from build123d import *

# Parameters (mm, degrees)
F1_DEPTH = 25
F3_DEPTH = 75
F4_W     = 5.629124
F4_H     = 6
F5_DEPTH = 35
F6_W     = 6.780945
F6_H     = 9.562873
F7_DEPTH = 3
F8_W     = 2
F8_H     = 9.562873
F9_DEPTH = 6


with BuildPart() as f1:
    # F0 (on Top) → F1 (new body)
    with BuildSketch(Plane.XY):
        with BuildLine():
            Line((-4.536292, 28.185949), (-55.529496, 19.979021))
            ThreePointArc((-55.529496, 19.979021), (-73.186468, 0), (-55.529496, -19.979021))
            Line((-55.529496, -19.979021), (-4.536292, -28.185949))
            ThreePointArc((-4.536292, -28.185949), (28.548654, 0), (-4.536292, 28.185949))
        make_face()
    extrude(amount=F1_DEPTH)

    # F2 (on face) → F3 (join)
    with BuildSketch(Plane.XY.offset(25)):
        Polygon((-10, 4.142136), (-10, -4.142136), (-4.142136, -10), (4.142136, -10), (10, -4.142136), (10, 4.142136), (4.142136, 10), (-4.142136, 10), align=None)
    extrude(amount=F3_DEPTH)

    # F4 (on face) → F5 (join)
    with BuildSketch(Plane.YZ.offset(10)):
        with Locations((-0.144606, 92.806667)):
            Rectangle(F4_W, F4_H)
    extrude(amount=F5_DEPTH)

    # F6 (on Front) → F7 (join, symmetric)
    with BuildSketch(Plane.XZ):
        with Locations((46.465266, 93.107711)):
            Rectangle(F6_W, F6_H)
    extrude(amount=F7_DEPTH, both=True)

    # F8 (on face) → F9 (cut)
    with BuildSketch(Plane.YZ.offset(49.855739)):
        with Locations((-0.098561, 93.107711)):
            Rectangle(F8_W, F8_H)
    extrude(amount=-F9_DEPTH, mode=Mode.SUBTRACT)


solid = f1.part
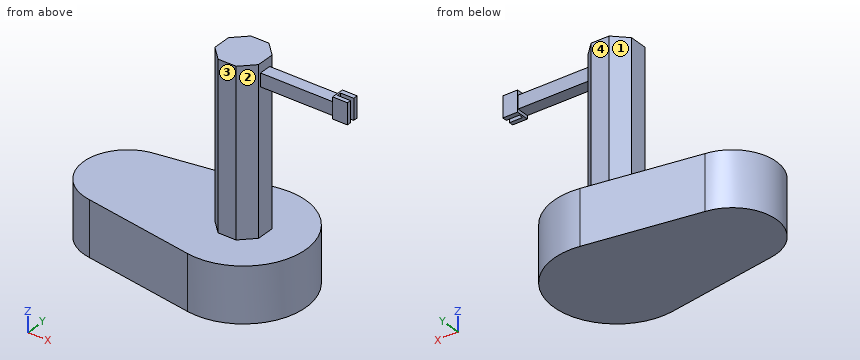
Build history of the part. All positions in model axes, mm. Face numbers are marked on the shaded views. A direction names the side the tool comes from. Give positions to 0.01 mm unless a question says otherwise; leave off trailing zeros. Order: outer loops, then holes, each group sorted by start corner. A loop starts at its lowest first (then second) coordinate and runs counter-clockwise, first axis right, second up. Notation, with made-up numbers: M 54,23 L 69,23 A19 ccw 69,39 Z; hole C 72,8 d10. An arc over 180 degrees is marked long. Use one line per item in the form item = value.
1) Drop flat-ended pins along their axis: pin 1 (4 mm diameter, centred on y = 1.5, z = 57.5, fed in from +X); pin 2 (9 mm diameter, centred on y = 1, z = 80.5, fed in from -X); pin 3 (6.5 mm diameter, centred on x = 32, z = 93, fed in from -Y). Give the stop position or say it passes through.
Calculated:
pin_1 = 10
pin_2 = -10
pin_3 = -2.96
2) Saw through at B-B (z = 29.5). Give the cut face in (x, y).
Calculated:
outline = M -10,-4.14 L -4.14,-10 L 4.14,-10 L 10,-4.14 L 10,4.14 L 4.14,10 L -4.14,10 L -10,4.14 Z
3) Tool access for the marked faces 1, 2, 3 and 4: list every direction of +Z, -Z, +X, -X, +Y, -Y with a clear straight run to the whole face (end or side of a thin tool).
Calculated:
face_1 = +Z, -X, +Y
face_2 = +Z, +X, -Y
face_3 = +Z, +X, -X, -Y
face_4 = +Z, +X, -X, +Y
4) Probe probe 1 along Z at (x, y) = (2.5, 12); probe 2 along Y at (x, z) = (-2, 95.5); probe 3 along Y at (x, z) = (44, 90.5). List the from-to ranges inside material, lowest first.
Calculated:
probe_1 = 0 to 25
probe_2 = -10 to 10
probe_3 = -3 to -1.1, 0.9 to 3
5) Saw through at C-C (y = -22). Give the cut face in (x, z), plus the area to 3 significant figures.
Calculated:
outline = M -42.97,0 L 18.19,0 L 18.19,25 L -42.97,25 Z
area = 1,530 mm2
6) Saw through at D-D (x = 34). Give the cut face in (y, z), plus the area to 3 significant figures.
Calculated:
outline = M -2.96,89.81 L 2.67,89.81 L 2.67,95.81 L -2.96,95.81 Z
area = 33.8 mm2
7) Saw through at A-A (x = 0). Give the cut face in (y, z), plus the area to 3 significant figures.
Calculated:
outline = M -28.55,0 L 28.55,0 L 28.55,25 L 10,25 L 10,100 L -10,100 L -10,25 L -28.55,25 Z
area = 2,930 mm2
